from build123d import *

# Parameters (mm, degrees)
SKETCH_1_R          = 55
SKETCH_1_R_2        = 1.5
SKETCH_1_R_3        = 6.5
EXTRUDE_1_DEPTH     = 2
SKETCH_3_R          = 2.25
CUT_EXTRUDE_1_DEPTH = 78.807454656


with BuildPart() as part:
    # 草图1 → 凸台-拉伸1 (new body)
    with BuildSketch(Plane.XY):
        Circle(SKETCH_1_R)
        with Locations((37.3, 15.5)):
            Circle(SKETCH_1_R_2, mode=Mode.SUBTRACT)
        with Locations((50.723393759, 7.75)):
            Circle(SKETCH_1_R_2, mode=Mode.SUBTRACT)
        with Locations((50.723393759, -7.75)):
            Circle(SKETCH_1_R_2, mode=Mode.SUBTRACT)
        with Locations((37.3, -15.5)):
            Circle(SKETCH_1_R_2, mode=Mode.SUBTRACT)
        with Locations((23.876606241, -7.75)):
            Circle(SKETCH_1_R_2, mode=Mode.SUBTRACT)
        with Locations((23.876606241, 7.75)):
            Circle(SKETCH_1_R_2, mode=Mode.SUBTRACT)
        Circle(SKETCH_1_R_3, mode=Mode.SUBTRACT)
        with BuildLine():
            Line((37.3, -6), (30, -6))
            ThreePointArc((30, -6), (24, 0), (30, 6))
            Line((30, 6), (37.3, 6))
            ThreePointArc((37.3, 6), (43.3, 0), (37.3, -6))
        make_face(mode=Mode.SUBTRACT)
    extrude(amount=EXTRUDE_1_DEPTH)

    # 草图3 → 切除-拉伸1 (cut, through all)
    with BuildSketch(Plane.XY.offset(2)):
        with Locations((0, 50)):
            Circle(SKETCH_3_R)
        with Locations((43.301270189, -25)):
            Circle(SKETCH_3_R)
        with Locations((-43.301270189, -25)):
            Circle(SKETCH_3_R)
    extrude(amount=-CUT_EXTRUDE_1_DEPTH, mode=Mode.SUBTRACT)


solid = part.part
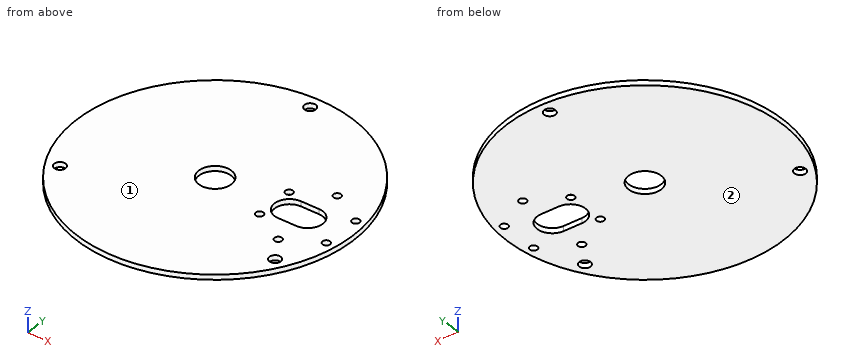
CAD build for the part. Positions are in the model's coordinates, mm. Face numbers are marked on the shaded views. Round coordinates to 2 decimals unless told otherwise and drop trailing zeros. Write each loop counter-clockwise with the first axis right and the second up, starting at its lowest first coordinate (ties: lowest second). Pieces come first, ordered by that corner, then holes. Notation, with made-up numbers: (41, 61.5) -> (46, 61.5) arc R16 cw to (46, 69.5) -> close; hole circle Ø1 at (-38.75, 48.5). An arc over 180 degrees is marked (long way). Answer as a JSON object with one key per item and string values.
(1) Pin check, flat tips, straight feed: P1, Ø4, axis at x = 37.3, y = -15.5, coming from the -Z side; P2, Ø4, axis at x = 43.3, y = -25, coming from the -Z side; P3, Ø1, axis at x = 24, z = 1.5, coming from the +Y side. Stop position of each tip, or through.
Reported:
{"P1": "stops at z = 0", "P2": "passes through", "P3": "stops at y = 49.73"}
(2) Probe probe 1 along Y at (x, z) = (0, 1.1); probe 2 along Y at (x, z) = (37.3, 1.2); probe 3 along Y at (x, z) = (2, 1.55). List the from-to ranges inside material, lowest first. Write a range as [from, to].
Reported:
{"probe 1": "y = [-55, -6.5], [6.5, 47.75], [52.25, 55]", "probe 2": "y = [-40.42, -17], [-14, -6], [6, 14], [17, 40.42]", "probe 3": "y = [-54.96, -6.18], [6.18, 48.97], [51.03, 54.96]"}
(3) Band-saw the part on B-B, the plane y = -15.5. List the corners of the cut face in (x, z).
Reported:
{"outline": "(-52.77, 0) -> (35.8, 0) -> (35.8, 2) -> (-52.77, 2) -> close; (38.8, 0) -> (52.77, 0) -> (52.77, 2) -> (38.8, 2) -> close"}
(4) Band-saw the part on A-A, the plane x = 33.5. List the corners of the cut face in (y, z).
Reported:
{"outline": "(-43.62, 0) -> (-6, 0) -> (-6, 2) -> (-43.62, 2) -> close; (6, 0) -> (43.62, 0) -> (43.62, 2) -> (6, 2) -> close"}
(5) Band-saw the part on C-C, the plane z = 0.9. Count the separate pieces of the cut face and the enclosed holes in it, then the cut area to 3 significant figures.
Reported:
{"separate pieces": "1", "enclosed holes": "11", "area": "9,080 mm^2"}
(6) Band-saw the part on D-D, the plane y = 7.75. List the corners of the cut face in (x, z), then the cut area to 3 significant figures.
Reported:
{"outline": "(-54.45, 0) -> (22.38, 0) -> (22.38, 2) -> (-54.45, 2) -> close; (25.38, 0) -> (49.22, 0) -> (49.22, 2) -> (25.38, 2) -> close; (52.22, 0) -> (54.45, 0) -> (54.45, 2) -> (52.22, 2) -> close", "area": "206 mm^2"}
(7) Two-plate mould, pull along Z, no slides. Class the marked faces 1 and 2: +Z half, -Z half, draft (parallel to the pull), parting line (faces both ways), or undercut.
Reported:
{"face 1": "+Z half", "face 2": "-Z half"}
